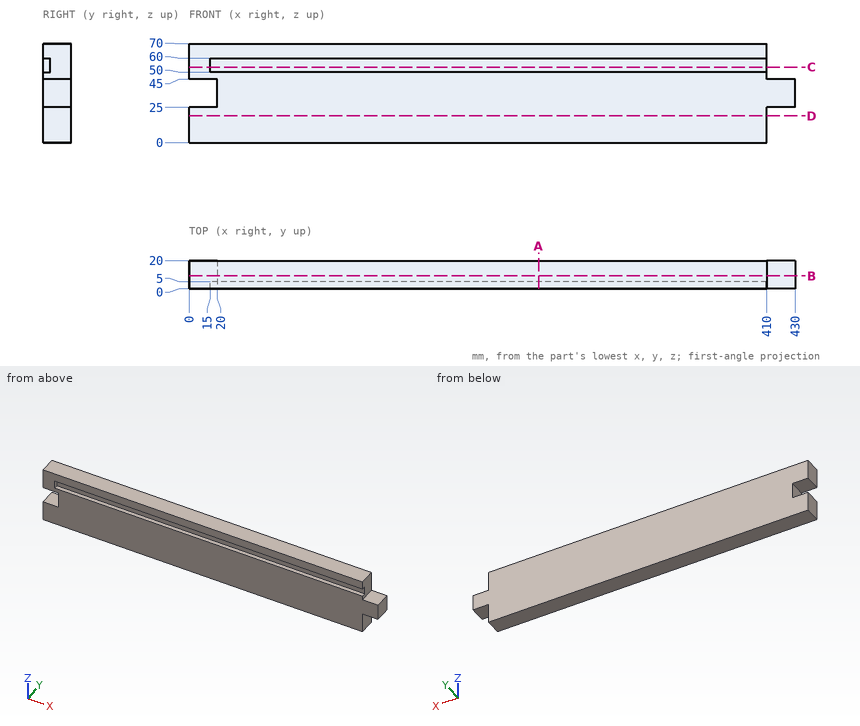
Print and shaded views of the part. All mm, measured from the part's lowest x, y and z. Coordinates: 2 decimals unless noted, no trailing zeros. Write each loop counter-clockwise with the first axis right and the second up, starting at its lowest first coordinate (ties: lowest second). Pieces come first, ordered by that corner, then holes.
(1) Cut at A-A, the plane x = 248. List the corners of the cut face in (y, z), and give its area (3 significant figures).
(2) Cut at D-D, the plane z = 19. List the corners of the cut face in (x, y), and give its area (3 significant figures).
(3) Flat gauge pins, fed straight in: pin 1 (12 mm diameter, centred on y = 14, z = 10, fed in from +X); pin 2 (6 mm diameter, centred on x = 424, y = 10.5, fed in from -Z); pin 3 (4 mm diameter, centred on y = 2.5, z = 53, fed in from +X). Where does each tip first touch, or does it go through?
(4) Cut at C-C, the plane z = 53.5. List the corners of the cut face in (x, y), and give its area (4 significant figures).
(5) Cut at B-B, the plane y = 9.25. List the corners of the cut face in (x, z), and give its area (3 significant figures).
(6) Drill centre lines: probe 1 along X at (y, z) = (17.25, 12); probe 2 along Z at (x, y) = (216, 3.25); probe 3 along X at (y, z) = (12, 36). Where is each one in solid material? Low to high.
Geometry says:
1. outline: (0, 0) - (20, 0) - (20, 70) - (0, 70) - (0, 60) - (5, 60) - (5, 50) - (0, 50) - close
1. area: 1,350 mm2
2. outline: (0, 0) - (410, 0) - (410, 20) - (0, 20) - close
2. area: 8,200 mm2
3. pin 1: stops at x = 410
3. pin 2: stops at z = 25
3. pin 3: stops at x = 15
4. outline: (0, 0) - (15, 0) - (15, 5) - (410, 5) - (410, 20) - (0, 20) - close
4. area: 6,225 mm2
5. outline: (0, 0) - (410, 0) - (410, 25) - (430, 25) - (430, 45) - (410, 45) - (410, 70) - (0, 70) - (0, 45) - (20, 45) - (20, 25) - (0, 25) - close
5. area: 28,700 mm2
6. probe 1: x = 0 to 410
6. probe 2: z = 0 to 50, 60 to 70
6. probe 3: x = 20 to 430
